from build123d import *

# Parameters (mm, degrees)
SALIENTE_EXTRUIR1_DEPTH = 1
CROQUIS2_R              = 4
SALIENTE_EXTRUIR2_DEPTH = 10


with BuildPart() as part:
    # Croquis1 → Saliente-Extruir1 (new body)
    with BuildSketch(Plane.XY):
        Polygon((0, -8.082903769), (7, -4.041451884), (7, 4.041451884), (0, 8.082903769), (-7, 4.041451884), (-7, -4.041451884), align=None)
    extrude(amount=SALIENTE_EXTRUIR1_DEPTH)

    # Croquis2 → Saliente-Extruir2 (add)
    with BuildSketch(Plane.XY.offset(1)):
        Circle(CROQUIS2_R)
    extrude(amount=SALIENTE_EXTRUIR2_DEPTH)

    # Croquis3 → Revolución1 (revolve)
    with BuildSketch(Plane(origin=(0, 0, 0), x_dir=(1, 0, 0), z_dir=(0, 1, 0))):
        Polygon((0, 21.382125591), (0.894479356, 21.382125591), (3.5, 17.682529237), (3.5, 16.666829395), (3, 16.666829395), (3, 15.620463348), (3.5, 15.620463348), (3.5, 11.644272372), (3, 11.644272372), (3, 10.737421798), (3.5, 10.737421798), (3.5, 6.900746294), (3, 6.900746294), (3, 5.784622511), (3.5, 5.784622511), (3.5, 2.645524372), (5.467415644, 2.645524372), (5.467415644, 1.808431535), (6.483115486, 1.808431535), (7, 0), (0, 0), align=None)
    revolve(axis=Axis((0, 0, 0), (0, 0, -1)))


solid = part.part
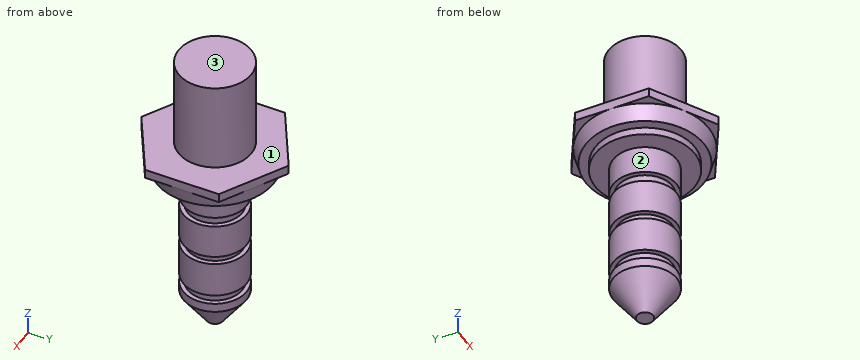
Read the model definition and answer for the solid it produces. Units are mm, in the model's axes. Face numbers are marked on the shaded views. A direction names the side the tool comes from. Round coordinates to 2 decimals unless told otherwise and drop trailing zeros. Loops run counter-clockwise (first coordinate to the right, second up) from the corner with the lowest first, then second, coordinate; pieces in that order, holes last. Notation, with made-up numbers: (-19.5, -10) - (23.5, -10) arc R14 cw to (23.5, 4) - close; hole circle Ø8 at (81.25, -29). An arc over 180 degrees is marked (long way). One line per question, with ' | ' between items. Start each with the question number.
Q1. For the marked faces 1, 2 and 3, determine the directions among +Z, -Z, +X, -X, +Y, -Y from which every point of the face is accessible in a straight line to the end or side of a thin tool.
Q2. Section B-B on z = -18 is taken. Give the vertices of the cut face in (x, y).
Q3. Section A-A on z = -9 is taken. Give the vertices of the cut face in (x, y), plus the area to 3 significant figures.
Q4. Flat-ended cylindrical pins translate along their axes: pin 1 (5 mm diameter, centred on y = -5, z = -7.5, fed in from -X); pin 2 (3 mm diameter, centred on x = -5, y = 3.5, fed in from -Z); pin 3 (2 mm diameter, centred on x = 0.5, y = -6.5, fed in from -Z). Find the tip coordinate at first contact, or state that the pin passes through.
Q5. Find the intervals of material crossed by L1, parallel to Z at x = -3.75, y = 2.75; L2, parallel to Z at x = -1.25, y = 3.75; L3, parallel to X at y = 1.75, z = -13, in increasing order.
Established:
1) face 1: +Z | face 2: -Z | face 3: +Z, +X, -X, +Y, -Y
2) outline: circle Ø6.55 at (0, 0)
3) outline: circle Ø7 at (0, 0) | area: 38.5 mm²
4) pin 1: x = -2.45 | pin 2: z = -2.65 | pin 3: z = -1.81
5) L1: -2.65 to 1 | L2: -2.65 to 11 | L3: -3.03 to 3.03
